Autodesk Inventor part; units mm, degrees
ref_plane "YZ Plane" through (0, 0, 0) normal (1, 0, 0) x (0, 1, 0)
ref_plane "XZ Plane" through (0, 0, 0) normal (0, 1, 0) x (-1, 0, 0)
ref_plane "XY Plane" through (0, 0, 0) normal (0, 0, 1) x (1, 0, 0)
sketch "Sketch1" plane through (0, 0, 0) normal (0, 1, 0) x (-1, 0, 0)
  circle A0 centre (0, 0) radius 19.5
  circle A1 centre (0, 0) radius 24.5
  dimension "d0" = 39
  dimension "d1" = 49
extrude "Extrusion1" add sketch "Sketch1" along normal blind 16
sketch "Sketch4" plane through (0, 16, 0) normal (0, 1, 0) x (1, 0, 0)
  circle A0 centre (0, 0) radius 24.5
  circle A1 centre (0, 0) radius 24.5
extrude "Extrusion3" add sketch "Sketch4" along normal blind 5
sketch "Sketch5" plane through (0, 16, 0) normal (0, -1, 0) x (1, 0, 0)
  circle A0 centre (0, 0) radius 8.75
  circle A1 centre (0, 0) radius 19.5
  dimension "d8" = 17.5
extrude "Extrusion4" add sketch "Sketch5" along normal blind 9
sketch "Sketch6" plane through (0, 7, 0) normal (0, -1, 0) x (1, 0, 0)
  circle A0 centre (0, 0) radius 19.5
  line L0 (-19.0853, 4) -> (19.0853, 4)
  line L1 (19.0853, 4) -> (19.0853, -4)
  line L2 (19.0853, -4) -> (-19.0853, -4)
  line L3 (-19.0853, -4) -> (-19.0853, 4)
  line L4 (-19.0853, 4) -> (19.0853, -4) construction
  line L5 (19.0853, 4) -> (-19.0853, -4) construction
  dimension "d11" = 8
extrude "Extrusion5" cut sketch "Sketch6" against normal blind 6 contours A0 L1 | L1 L2 L3 L0 | L3 A0
sketch "Sketch7" plane through (0, 16, 0) normal (0, -1, 0) x (1, 0, 0)
  circle A0 centre (0, 0) radius 4.125
  dimension "d14" = 8.25
extrude "Extrusion6" cut sketch "Sketch7" against normal blind 5
properties part number "SeguroRueda"
Input: part model. Units: mm. Frame: model coordinates. A direction names the side the tool comes from. Round coordinates to 2 decimals unless told otherwise and drop trailing zeros. Loops run counter-clockwise (first coordinate to the right, second up) from the corner with the lowest first, then second, coordinate; pieces in that order, holes last. Notation, with made-up numbers: (16.25, -38.5) - (46.25, -38.5) arc R20 cw to (46.25, -29.5) - close; hole circle Ø11 at (-18.75, 7.5). An arc over 180 degrees is marked (long way). One line per item, written item: value. Start each with the question number.
(1) Contact query for flat-ended pins moving along their axis: P1, Ø1, axis at x = -15.5, z = 8, coming from the -Y side; P2, Ø4, axis at x = 15.5, y = 3.5, coming from the +Z side; P3, Ø8, axis at x = 11.5, y = 15.5, coming from the -Z side. Output: stop coordinate, or through.
(2) Section C-C, the plane z = -11. Return loops of the section in (x, y), plus the area to 3 significant figures.
(3) Section D-D, the plane y = 6. Return loops of the section in (x, z), plus the area to 3 significant figures.
(4) Access query for faces 3 (the flat face through (16.45, 0, -10.77)), 4 (the cylindrical face through (-13.17, 4.96, -14.38)). Directions: +Z, -Z, +X, -X, +Y, -Y. A direction counts if a zero-diameter tool reaches every point of the face in a straight line with its end or side. Return the directions, or none.
(5) Ray query, line 1 (Z direction, x = 0, y = 12.5); line 2 (Z direction, x = 0, y = 18.8) (3 decimals); line 3 (X direction, y = 11.75, z = 0). Return the intervals inside material, ascending. Write a range as [from, to].
(6) Draft query along X for faces 1 (the flat face through (-14, 10, 4)), 2 (the flat face through (5, 21, 0)). Return one class per face: +X half, -X half, draft (parallel to the pull), parting line (faces both ways), or undercut.
(7) Section A-A, the plane y = 10.75. Return loops of the section in (x, z), plus the area to 3 significant figures.
Results below:
1. P1: y = 7
1. P2: z = 20.45
1. P3: z = -23.32
2. outline: (-21.89, 0) - (-16.1, 0) - (-16.1, 7) - (16.1, 7) - (16.1, 0) - (21.89, 0) - (21.89, 21) - (-21.89, 21) - close
2. area: 694 mm^2
3. outline: circle Ø49 at (0, 0); hole circle Ø39 at (0, 0)
3. area: 691 mm^2
4. face 3: +Z, -Z, +X, -X, -Y
4. face 4: -Y
5. line 1: [-24.5, -8.75], [8.75, 24.5]
5. line 2: [-24.5, -4.125], [4.125, 24.5]
5. line 3: [-24.5, -19.5], [19.5, 24.5]
6. face 1: undercut
6. face 2: draft
7. outline: circle Ø49 at (0, 0); hole (-19.09, -4) - (-7.78, -4) arc R8.75 ccw to (7.78, -4) - (19.09, -4) arc R19.5 ccw to (19.09, 4) - (7.78, 4) arc R8.75 ccw to (-7.78, 4) - (-19.09, 4) arc R19.5 ccw to start
7. area: 1,470 mm^2
